The listing builds one solid part. Answer for the finished solid, in the listing's coordinates (mm). A direction names the side the tool comes from. Round coordinates to 2 decimals unless told otherwise and drop trailing zeros. Order: outer loops, then holes, each group sorted by start corner. A loop starts at its lowest first (then second) coordinate and runs counter-clockwise, first axis right, second up. Notation, with made-up numbers: (89, 35) -> (141, 35) arc R20 ccw to (141, 41) -> close; hole circle Ø9 at (-33, 72). An arc over 180 degrees is marked (long way). Return JSON: item names as keys, results as strings. Group by question number.
(1) The part is cut by section D-D (z = 3.7). Determine the outline of the cut face in (x, y) (3 decimals).
(2) The part is cut by section A-A (z = 1.4). Determine the outline of the cut face in (x, y) (3 decimals).
(3) Consider line 1 (Y direction, x = 15.1, z = 2.85) (3 decimals); line 2 (X direction, y = 6.5, z = 0.9); line 3 (Y direction, x = 7.55, z = 3.15). Determine where each line is inside the solid, lowest interval first. Write a range as [from, to].
(4) Determine the mould class of faces 4 (the face through (17.772, 9.072, 0.986)), 5 (the face through (0, 7, 2)), 6 (the face through (24, 6, 2)), 7 (the face through (28.997, 13.859, 2.028)) for opening direction X: +X half, -X half, draft (parallel to the pull), parting line (faces both ways), or undercut.
(5) The part is cut by section C-C (y = 8). Determine the outline of the cut face in (x, z).
(6) The part is cut by section B-B (x = 7.55). Determine the outline of the cut face in (y, z) (3 decimals).
(7) Each of these flat-tipped pins is pushed along its axis until it touches: pin 1 (3.5 mm diameter, centred on x = 22.5, y = 7.5, fed in from +Z); pin 2 (2 mm diameter, centred on x = 21.5, y = 13, fed in from -Z); pin 3 (1.7 mm diameter, centred on x = 15, y = 8, fed in from +Z). Where does it stop, or does it pass through?
(8) Which of the six approach directions +Z, -Z, +X, -X, +Y, -Y give full straight-line access (tool end or side, diameter ignored) to faces 1 (the face through (16.027, 8.955, 3.138)), 2 (the face through (15, 4.4, 1)), 3 (the face through (15, 0, 2))?
from build123d import *

# Parameters (mm, degrees)
F0_W     = 30.2
F0_H     = 15
F0_R     = 1.725
F1_DEPTH = 4
F2_R     = 3.5
F3_DEPTH = 2
F5_DEPTH = 2
F6_R     = 1.75
F7_DEPTH = 0.3
F8_R     = 4


with BuildPart() as f1:
    # F0 (on Top) → F1 (new body)
    with BuildSketch(Plane.XY):
        with Locations((15.1, 7.5)):
            Rectangle(F0_W, F0_H)
        with Locations((7.55, 7.5)):
            Circle(F0_R, mode=Mode.SUBTRACT)
        with Locations((15.1, 7.5)):
            Circle(F0_R, mode=Mode.SUBTRACT)
        with Locations((22.65, 7.5)):
            Circle(F0_R, mode=Mode.SUBTRACT)
    extrude(amount=F1_DEPTH)

    # F2 (on face) → F3 (cut)
    with BuildSketch(Plane.XY.offset(4)):
        with Locations((7.55, 7.5)):
            Circle(F2_R)
        with Locations((22.65, 7.5)):
            Circle(F2_R)
    extrude(amount=-F3_DEPTH, mode=Mode.SUBTRACT)

    # F4 (on face) → F5 (cut)
    with BuildSketch(Plane(origin=(0, 0, 0), x_dir=(1, 0, 0), z_dir=(0, 0, -1))):
        Polygon((18.679572, -7.5), (16.889786, -4.4), (13.310214, -4.4), (11.520428, -7.5), (13.310214, -10.6), (16.889786, -10.6), align=None)
    extrude(amount=-F5_DEPTH, mode=Mode.SUBTRACT)

    # F6 (on face) → F7 (join)
    with BuildSketch(Plane(origin=(0, 0, 2), x_dir=(1, 0, 0), z_dir=(0, 0, -1))):
        with Locations((15.1, -7.5)):
            Circle(F6_R)
    extrude(amount=-F7_DEPTH)

    # F8
    f8_edges = [f1.edges().sort_by_distance(p)[0] for p in [
        (0, 0, 2),
        (30.2, 0, 2),
        (30.2, 15, 2),
        (0, 15, 2),
    ]]
    fillet(f8_edges, radius=F8_R)


solid = f1.part
Answer below:
{
 "1": {"outline": "(0, 4) arc R4 ccw to (4, 0) -> (26.2, 0) arc R4 ccw to (30.2, 4) -> (30.2, 11) arc R4 ccw to (26.2, 15) -> (4, 15) arc R4 ccw to (0, 11) -> close; hole circle Ø7 at (7.55, 7.5); hole circle Ø3.45 at (15.1, 7.5); hole circle Ø7 at (22.65, 7.5)"},
 "2": {"outline": "(0, 4) arc R4 ccw to (4, 0) -> (26.2, 0) arc R4 ccw to (30.2, 4) -> (30.2, 11) arc R4 ccw to (26.2, 15) -> (4, 15) arc R4 ccw to (0, 11) -> close; hole circle Ø3.45 at (7.55, 7.5); hole (11.52, 7.5) -> (13.31, 4.4) -> (16.89, 4.4) -> (18.68, 7.5) -> (16.89, 10.6) -> (13.31, 10.6) -> close; hole circle Ø3.45 at (22.65, 7.5)"},
 "3": {"line 1": "y = [0, 5.775], [9.225, 15]", "line 2": "x = [0, 6.14], [8.96, 12.1], [18.1, 21.24], [24.06, 30.2]", "line 3": "y = [0, 4], [11, 15]"},
 "4": {"face 4": "undercut", "face 5": "-X half", "face 6": "undercut", "face 7": "+X half"},
 "5": {"outline": "(0, 0) -> (5.9, 0) -> (5.9, 2) -> (4.09, 2) -> (4.09, 4) -> (0, 4) -> close; (9.2, 0) -> (11.81, 0) -> (11.81, 2) -> (18.39, 2) -> (18.39, 0) -> (21, 0) -> (21, 2) -> (19.19, 2) -> (19.19, 4) -> (16.75, 4) -> (16.75, 2.3) -> (13.45, 2.3) -> (13.45, 4) -> (11.01, 4) -> (11.01, 2) -> (9.2, 2) -> close; (24.3, 0) -> (30.2, 0) -> (30.2, 4) -> (26.11, 4) -> (26.11, 2) -> (24.3, 2) -> close"},
 "6": {"outline": "(0, 0) -> (5.775, 0) -> (5.775, 2) -> (4, 2) -> (4, 4) -> (0, 4) -> close; (9.225, 0) -> (15, 0) -> (15, 4) -> (11, 4) -> (11, 2) -> (9.225, 2) -> close"},
 "7": {"pin 1": "stops at z = 2", "pin 2": "stops at z = 0", "pin 3": "stops at z = 2.3"},
 "8": {"face 1": "+Z", "face 2": "-Z", "face 3": "+Z, -Z, +X, -X, -Y"}
}
